Could you check a few things on this model? Use its own coordinates, in mm. A direction names the side the tool comes from. Coordinates: 2 decimals unless noted, no trailing zeros. Write each loop counter-clockwise with the first axis right and the second up, starting at its lowest first coordinate (ties: lowest second). Pieces come first, ordered by that corner, then holes. Notation, with made-up numbers: (66, 85) - (105, 85) arc R24 ccw to (105, 119) - close; hole circle Ø5 at (41, 9.5). An arc over 180 degrees is marked (long way). Answer as a JSON object with one key per item and string values. Group by question number.
1) On a 3-axis mill with a long thin cutter (end or side, diameter ignored), from which of +Z, -Z, +X, -X, +Y, -Y can I reach the whole of each face in a straight line? I mean faces 4 (the flat face through (-22.34, 67, 1)), 5 (the flat face through (4, 35.566, 1)), 6 (the cylindrical face through (14.09, 20.17, 1.01)). Say none if no direction works.
2) Please list where these lines run through material, in increasing order: line 1 along Y through (x, z) = (-13.5, 0.35); line 2 along Y through (x, z) = (-6, 1.9); line 3 along Y through (x, z) = (-3, 0.6).
3) If we section it at A-A (x = 0): Write out the boundary of the cut face in (y, z), plus the area to 3 significant figures.
4) Will these pins go through, and if not, where does the flat tip stop? pin 1 Ø5 at (x, y) = (-33.34, 27.57) entering from +Z; pin 2 Ø0.6 at (x, z) = (-32, 1) entering from +Y; pin 3 Ø1 at (y, z) = (58, 0.5) entering from -X; pin 4 Ø0.6 at (x, z) = (0, 1.5) entering from +Y.
5) If we section it at D-D (y = 58.5): Write out the boundary of the cut face in (x, z).
6) If we section it at B-B (z = 0.4): State how many separate pieces and enclosed holes the cut face has, plus the area to 3 significant figures.
7) We'd pull the mould along Y, two halves only. Please class faces 1 (the flat face through (14.66, 27, 1)), 2 (the flat face through (-14, 19.566, 1)), 3 (the flat face through (-4.34, 66, 1)): released by +Y, released by -Y, zero draft, split by the parting line, or undercut.
8) If we section it at C-C (x = -21): Write out the boundary of the cut face in (y, z), plus the area to 3 significant figures.
```python
from build123d import *

# Parameters (mm, degrees)
SKETCH_1_R      = 2
SKETCH_1_R_2    = 2.05
EXTRUDE_1_DEPTH = 2
FILLET_1_R      = 2


with BuildPart() as part:
    # 草图1 → 凸台-拉伸1 (new body)
    with BuildSketch(Plane.XY):
        with BuildLine():
            Line((14.659550972, 19.565520938), (14.659550972, 35.565520938))
            Line((14.659550972, 35.565520938), (-4.340449028, 35.565520938))
            Line((-4.340449028, 35.565520938), (-4.340449028, 96.97706367))
            ThreePointArc((-4.340449028, 96.97706367), (-13.340449028, 130.565520938), (-22.340449028, 96.97706367))
            Line((-22.340449028, 96.97706367), (-22.340449028, 35.565520938))
            Line((-22.340449028, 35.565520938), (-41.340449028, 35.565520938))
            Line((-41.340449028, 35.565520938), (-41.340449028, 19.565520938))
            Line((-41.340449028, 19.565520938), (14.659550972, 19.565520938))
        make_face()
        with Locations((-33.340449028, 27.565520938)):
            Circle(SKETCH_1_R, mode=Mode.SUBTRACT)
        with Locations(Location((6.659550972, 27.565520938, 0), (0, 0, 180))):
            Circle(SKETCH_1_R, mode=Mode.SUBTRACT)
        with Locations((-13.340449028, 112.565520938)):
            Circle(SKETCH_1_R, mode=Mode.SUBTRACT)
        with Locations((-13.340449028, 47.565520938)):
            Circle(SKETCH_1_R, mode=Mode.SUBTRACT)
        with Locations((-4.840449028, 121.065520938)):
            Circle(SKETCH_1_R_2, mode=Mode.SUBTRACT)
        with Locations((-4.840449028, 104.065520938)):
            Circle(SKETCH_1_R_2, mode=Mode.SUBTRACT)
        with Locations((-21.840449028, 104.065520938)):
            Circle(SKETCH_1_R_2, mode=Mode.SUBTRACT)
        with Locations((-21.840449028, 121.065520938)):
            Circle(SKETCH_1_R_2, mode=Mode.SUBTRACT)
    extrude(amount=EXTRUDE_1_DEPTH)

    # 圆角1
    fillet_1_edges = [part.edges().sort_by_distance(p)[0] for p in [
        (-41.340449028, 19.565520938, 1),
        (-41.340449028, 35.565520938, 1),
        (14.659550972, 35.565520938, 1),
        (14.659550972, 19.565520938, 1),
    ]]
    fillet(fillet_1_edges, radius=FILLET_1_R)


solid = part.part
```
Here are the results:
{
 "1": {"face 4": "+Z, -Z, -X", "face 5": "+Z, -Z, +X", "face 6": "+Z, -Z, +X, -Y"},
 "2": {"line 1": "y = 19.57 to 45.57, 49.56 to 110.57, 114.56 to 130.56", "line 2": "y = 19.57 to 102.37, 105.76 to 119.37, 122.76 to 129", "line 3": "y = 19.57 to 35.57, 97.83 to 103.16, 104.97 to 120.16, 121.97 to 127.3"},
 "3": {"outline": "(19.57, 0) - (35.57, 0) - (35.57, 2) - (19.57, 2) - close; (100.48, 0) - (124.65, 0) - (124.65, 2) - (100.48, 2) - close", "area": "80.3 mm²"},
 "4": {"pin 1": "stops at z = 2", "pin 2": "stops at y = 35.57", "pin 3": "stops at x = -22.34", "pin 4": "stops at y = 124.97"},
 "5": {"outline": "(-22.34, 0) - (-4.34, 0) - (-4.34, 2) - (-22.34, 2) - close"},
 "6": {"separate pieces": "1", "enclosed holes": "8", "area": "2,880 mm²"},
 "7": {"face 1": "zero draft", "face 2": "released by -Y", "face 3": "undercut"},
 "8": {"outline": "(19.57, 0) - (102.2, 0) - (102.2, 2) - (19.57, 2) - close; (105.94, 0) - (119.2, 0) - (119.2, 2) - (105.94, 2) - close; (122.94, 0) - (128.85, 0) - (128.85, 2) - (122.94, 2) - close", "area": "204 mm²"}
}
